```python
from build123d import *

# Parameters (mm, degrees)
SKICA1_W                = 350
SKICA1_H                = 650
P_IDAT_VYSUNUT_M2_DEPTH = 18


with BuildPart() as part:
    # Skica1 → Přidat vysunutím2 (new body)
    with BuildSketch(Plane.XY):
        with Locations((175, 325)):
            Rectangle(SKICA1_W, SKICA1_H)
    extrude(amount=P_IDAT_VYSUNUT_M2_DEPTH)

    # Odebrat tažením po křivce8: sweep along a path in cesta
    with BuildLine(Plane.XY.offset(18)) as odebrat_ta_en_m_po_k_ivce8_path:
        Line((175, 0), (175, 602.357194164))
        Line((175, 602.357194164), (68.787703731, 602.357194164))
    # profil na frezu → Odebrat tažením po křivce8 (sweep, cut)
    with BuildSketch(Plane.XZ):
        Polygon((190, 3), (190, 8), (177.5, 8), (177.5, 18), (172.5, 18), (172.5, 8), (160, 8), (160, 3), align=None)
    sweep(path=odebrat_ta_en_m_po_k_ivce8_path.line, transition=Transition.RIGHT, mode=Mode.SUBTRACT)


solid = part.part
```
Model file for the job. Use its own axes, mm. A direction names the side the tool comes from. Give positions to 0.01 mm unless a question says otherwise; leave off trailing zeros. Order: outer loops, then holes, each group sorted by start corner. A loop starts at its lowest first (then second) coordinate and runs counter-clockwise, first axis right, second up.
1) Pin check, flat tip, straight feed: pin 1 (6 mm diameter, centred on y = 180, z = 4.5, fed in from -X). Stop position of the tip, or through.
2) Saw through at C-C, the plane x = 91.5. Write the cut outline in (y, z).
3) Wall check: probe 1 along X at (y, z) = (254, 12); probe 2 along X at (y, z) = (603.5, 8.5); probe 3 along Z at (x, y) = (161, 243.5). Give the ranges that are in metal, low to high.
4) 3-axis set-ups, long thin cutter, end or side, ignore diameter. For faces 1 (the flat face through (0, 320, 9)), 2 (the flat face through (179, 379, 8)): which of +Z, -Z, +X, -X, +Y, -Y reach the whole face in a straight line?
5) Mould opens along Z. For faces 3 (the flat face through (68.788, 602, 7)), 4 (the flat face through (173, 330, 0)), 5 (the flat face through (173, 0, 1)), 6 (the flat face through (163, 368, 8)) say: +Z half, -Z half, draft (parallel to the pull), parting line (faces both ways), or undercut.
6) Saw through at B-B, the plane z = 13.75. Write the cut outline in (x, y), then the cut area to 3 significant figures.
7) Saw through at A-A, the plane y = 423. Write the cut outline in (x, z).
Computed:
1. pin 1: stops at x = 0
2. outline: (0, 0) - (650, 0) - (650, 18) - (604.86, 18) - (604.86, 8) - (617.36, 8) - (617.36, 3) - (587.36, 3) - (587.36, 8) - (599.86, 8) - (599.86, 18) - (0, 18) - close
3. probe 1: x = 0 to 172.5, 177.5 to 350
3. probe 2: x = 0 to 68.79, 177.5 to 350
3. probe 3: z = 0 to 3, 8 to 18
4. face 1: +Z, -Z, -X, +Y, -Y
4. face 2: none
5. face 3: undercut
5. face 4: -Z half
5. face 5: draft
5. face 6: undercut
6. outline: (0, 0) - (172.5, 0) - (172.5, 599.86) - (68.79, 599.86) - (68.79, 604.86) - (177.5, 604.86) - (177.5, 0) - (350, 0) - (350, 650) - (0, 650) - close
6. area: 224,000 mm2
7. outline: (0, 0) - (350, 0) - (350, 18) - (177.5, 18) - (177.5, 8) - (190, 8) - (190, 3) - (160, 3) - (160, 8) - (172.5, 8) - (172.5, 18) - (0, 18) - close
